Autodesk Fusion 360 part; units mm, degrees
sketch "Sketch1" plane through (0, 0, 0) normal (0, 0, 1) x (1, 0, 0) in component "WeCopy"
  line L0 (0, 0) -> (96.62, 0)
  line L1 (96.62, 0) -> (96.62, 23.86)
  line L2 (96.62, 23.86) -> (0, 23.86)
  line L3 (0, 23.86) -> (0, 0)
  line L4 (-9.5, -9.5) -> (106.12, -9.5)
  line L5 (106.12, -9.5) -> (106.12, 33.36)
  line L6 (106.12, 33.36) -> (-9.5, 33.36)
  line L7 (-9.5, 33.36) -> (-9.5, -9.5)
  circle A0 centre (101.12, 28.36) radius 1.7
  circle A1 centre (101.12, -4.5) radius 1.7
  circle A2 centre (-4.5, 28.36) radius 1.7
  circle A3 centre (-4.5, -4.5) radius 1.7
  circle A4 centre (101.12, 28.36) radius 3
  circle A5 centre (101.12, -4.5) radius 3
  circle A6 centre (-4.5, -4.5) radius 3
  circle A7 centre (-4.5, 28.36) radius 3
  dimension "d1" = 96.62
  dimension "d2" = 23.86
  dimension "d3" = 115.62
  dimension "d4" = 42.86
  dimension "d5" = 9.5
  dimension "d6" = 9.5
  dimension "d7" = 9.5
  dimension "d8" = 9.5
  dimension "d9" = 3.4
  dimension "d10" = 3.4
  dimension "d11" = 3.4
  dimension "d12" = 3.4
  dimension "d13" = 5
  dimension "d14" = 5
  dimension "d15" = 5
  dimension "d16" = 5
  dimension "d17" = 5
  dimension "d18" = 5
  dimension "d19" = 5
  dimension "d20" = 5
  dimension "d21" = 6
  dimension "d22" = 6
  dimension "d23" = 6
  dimension "d24" = 6
extrude "Extrude2" add sketch "Sketch1" along normal blind 9.9 from surface at 3.1 contours A4 | A5 | A6 | A7 makes body 1 at (99.7514, 25.6904, 6.4) makes body 2 at (-1.5037, -4.6495, 9.7) makes body 3 at (101.9325, -1.6121, 9.7) makes body 4 at (-1.5037, 28.2105, 9.7) in component "WeCopy"
extrude "Extrude3" add sketch "Sketch1" along normal blind 13 contours L4 L5 L6 L7 bodies 1 2 3 4 in component "WeCopy"
extrude "Extrude4" add sketch "Sketch1" along normal blind 3 contours L0 L1 L2 L3 bodies 1 in component "WeCopy"
sketch "Sketch2" plane through (0, 0, 3) normal (0, 0, 1) x (-1, 0, 0) in component "WeCopy"
  line L0 (0, -23.86) -> (0, 0)
  line L1 (0, 0) -> (-96.62, 0)
  line L2 (-96.62, 0) -> (-96.62, -23.86)
  line L3 (-96.62, -23.86) -> (0, -23.86)
  line L4 (14, -21.2325) -> (-4.5, -21.2325)
  line L5 (-4.5, -21.2325) -> (-4.5, -2.7325)
  line L6 (-4.5, -2.7325) -> (14, -2.7325)
  line L7 (14, -2.7325) -> (14, -21.2325)
  line L8 (9.5, 9.5) -> (-106.12, 9.5)
  dimension "d35" = 18.5
  dimension "d36" = 18.5
  dimension "d37" = 12.2325
extrude "Extrude5" cut sketch "Sketch2" against normal blind 7.5 from surface at 10 contours L0 L4 L6 L7 bodies 1 in component "WeCopy"
fillet "Fillet1" radius 5 1 edges at (-9.5, 33.36, 6.5) on bodies 1 in component "WeCopy"
fillet "Fillet2" radius 5 1 edges at (-9.5, -9.5, 6.5) on bodies 1 in component "WeCopy"
fillet "Fillet3" radius 5 1 edges at (106.12, -9.5, 6.5) on bodies 1 in component "WeCopy"
fillet "Fillet4" radius 5 1 edges at (106.12, 33.36, 6.5) on bodies 1 in component "WeCopy"
component "WeCopy" placed x (1, 0, 0) y (0, 1, 0) z (0, 0, 1) at (0, 0, 0)
Read the model definition and answer for the solid it produces. Units are mm, in the model's axes. A direction names the side the tool comes from. Give positions to 0.01 mm unless a question says otherwise; leave off trailing zeros. Order: outer loops, then holes, each group sorted by start corner. A loop starts at its lowest first (then second) coordinate and runs counter-clockwise, first axis right, second up. Notation, with made-up numbers: (20, -14) -> (50, -14) arc R27 ccw to (50, 9) -> close; hole circle Ø8 at (61, 1). An arc over 180 degrees is marked (long way). One line per item, written item: value. Start each with the question number.
(1) For a pull along Y with two mould halves and no side action, classify faces 4 (the flat face through (106.12, 12, 6)), 5 (the flat face through (101.1, -6.5, 3.1)), 6 (the flat face through (49, 33.36, 6)) as released by +Y, released by -Y, zero draft, split by the parting line, or undercut.
(2) A tool of negligible diameter and unlimited length cuts with its end or side. For faces 1 (the flat face through (96.62, 12, 8)), 2 (the cylindrical face through (98.123, -4.632, 1.528)), 3 (the flat face through (-5, 12, 5.5)), from which of +Z, -Z, +X, -X, +Y, -Y can it reach the whole face along a straight path? Write none if from no direction.
(3) The part is cut by section D-D (z = 8.75). Determine the outline of the cut face in (x, y), and give its area (3 significant figures).
(4) Straight lines are drawn through the part: L1, parallel to Y at x = 101.12, z = 2.2; L2, parallel to Y at x = 101.12, z = 7.75; L3, parallel to Y at x = 76.5, z = 7.75. For each, find the intervals that lie inside material, in ascending order.
(5) The part is cut by section B-B (y = 22.5). Determine the outline of the cut face in (x, z), and give its area (3 significant figures).
(6) The part is cut by section C-C (x = 77.5). Determine the outline of the cut face in (y, z), and give its area (3 significant figures).
(7) Flat-ended cylindrical pins translate along their axes: P1, Ø12, axis at x = 82.5, y = 20.5, coming from the -Z side; P2, Ø5.5, axis at x = -4.5, y = -4.5, coming from the -Z side; P3, Ø3, axis at x = -4, y = 10.5, coming from the +Z side; P4, Ø2, axis at x = 101.12, y = -4.5, coming from the -Z side. Find the tip coordinate at first contact, or state that the pin passes through.
(8) The part is cut by section A-A (z = 1.5). Determine the outline of the cut face in (x, y), and give its area (3 significant figures).
Taken from the geometry:
1. face 4: zero draft
1. face 5: undercut
1. face 6: released by +Y
2. face 1: +Z
2. face 2: -Z
2. face 3: +Z, -X
3. outline: (-9.5, -4.5) arc R5 ccw to (-4.5, -9.5) -> (101.12, -9.5) arc R5 ccw to (106.12, -4.5) -> (106.12, 28.36) arc R5 ccw to (101.12, 33.36) -> (-4.5, 33.36) arc R5 ccw to (-9.5, 28.36) -> (-9.5, 21.23) -> (0, 21.23) -> (0, 23.86) -> (96.62, 23.86) -> (96.62, 0) -> (0, 0) -> (0, 2.73) -> (-9.5, 2.73) -> close; hole circle Ø3.4 at (-4.5, -4.5); hole circle Ø3.4 at (-4.5, 28.36); hole circle Ø3.4 at (101.12, -4.5); hole circle Ø3.4 at (101.12, 28.36)
3. area: 2,420 mm^2
4. L1: -9.5 to -7.5, -1.5 to 25.36, 31.36 to 33.36
4. L2: -9.5 to -6.2, -2.8 to 26.66, 30.06 to 33.36
4. L3: -9.5 to 0, 23.86 to 33.36
5. outline: (-9.5, 0) -> (106.12, 0) -> (106.12, 13) -> (96.62, 13) -> (96.62, 3) -> (0, 3) -> (0, 13) -> (-9.5, 13) -> close
5. area: 537 mm^2
6. outline: (-9.5, 0) -> (33.36, 0) -> (33.36, 13) -> (23.86, 13) -> (23.86, 3) -> (0, 3) -> (0, 13) -> (-9.5, 13) -> close
6. area: 319 mm^2
7. P1: z = 0
7. P2: z = 3.1
7. P3: z = 5.5
7. P4: through
8. outline: (-9.5, -4.5) arc R5 ccw to (-4.5, -9.5) -> (101.12, -9.5) arc R5 ccw to (106.12, -4.5) -> (106.12, 28.36) arc R5 ccw to (101.12, 33.36) -> (-4.5, 33.36) arc R5 ccw to (-9.5, 28.36) -> close; hole circle Ø6 at (-4.5, -4.5); hole circle Ø6 at (-4.5, 28.36); hole circle Ø6 at (101.12, -4.5); hole circle Ø6 at (101.12, 28.36)
8. area: 4,820 mm^2
